Part model, mm, in its own coordinate system. A direction names the side the tool comes from. Coordinates: 2 decimals unless noted, no trailing zeros. Write each loop counter-clockwise with the first axis right and the second up, starting at its lowest first coordinate (ties: lowest second). Pieces come first, ordered by that corner, then holes. Notation, with made-up numbers: (56.5, -30.5) -> (104.5, -30.5) arc R28 cw to (104.5, -10.5) -> close; hole circle Ø10 at (51.25, 7.5). An arc over 180 degrees is marked (long way). Write item = value, one per line. Start each with the question number.
Q1. Band-saw the part on D-D, the plane x = 38.1. List the corners of the cut face in (y, z).
Q2. Tool access for faces 1 (the flat face through (25, 0, 17.462)), 2 (the flat face through (25, 0, 19.05)): list every direction of +Z, -Z, +X, -X, +Y, -Y with a clear straight run to the whole face (end or side of a thin tool).
Q3. Band-saw the part on B-B, the plane y = 3.25. List the corners of the cut face in (x, z), plus the area to 3 significant figures.
Q4. Band-saw the part on A-A, the plane z = 13. List the corners of the cut face in (x, y).
Q5. Probe line 1 (Y direction, x = 13.5, z = -15); line 2 (Z direction, x = 30.5, y = 0); line 3 (Z direction, x = 38.1, y = 12.05). List the from-to ranges inside material, lowest first.
Q6. Band-saw the part on C-C, the plane x = 18. List the corners of the cut face in (y, z), plus the area to 3 significant figures.
Q7. Pull direction Z, two halves, no side cores. Call faces 3 (the flat face through (25, -12.7, 0)), 4 (the flat face through (25, 0, -17.462)), 5 (the flat face through (25, 0, -19.05)): released by +Z, released by -Z, zero draft, split by the parting line, or undercut.
Autodesk Inventor part; units mm, degrees
ref_plane "Work Plane3" through (0, 12.7, 0) normal (0, 1, 0) x (-1, 0, 0)
ref_plane "Start Plane" through (0, 0, 0) normal (1, 0, 0) x (0, 1, 0)
ref_plane "End Plane" through (50.8, 0, 0) normal (1, 0, 0) x (0, 1, 0)
ref_plane "Work Plane3" through (0, 12.7, 0) normal (0, 1, 0) x (-1, 0, 0)
ref_plane "Start Plane" through (0, 0, 0) normal (1, 0, 0) x (0, 1, 0)
ref_plane "End Plane" through (50.8, 0, 0) normal (1, 0, 0) x (0, 1, 0)
sketch "Sketch" plane through (0, 0, 0) normal (1, 0, 0) x (0, 1, 0)
  line L0 (-12.7, 19.05) -> (12.7, 19.05)
  line L1 (12.7, 19.05) -> (12.7, -19.05)
  line L2 (12.7, -19.05) -> (-12.7, -19.05)
  line L3 (-12.7, -19.05) -> (-12.7, 19.05)
  line L4 (-12.7, 19.05) -> (12.7, -19.05) construction
  line L5 (12.7, 19.05) -> (-12.7, -19.05) construction
  line L6 (-11.1125, 17.4625) -> (11.1125, 17.4625)
  line L7 (11.1125, 17.4625) -> (11.1125, -17.4625)
  line L8 (11.1125, -17.4625) -> (-11.1125, -17.4625)
  line L9 (-11.1125, -17.4625) -> (-11.1125, 17.4625)
  line L10 (-11.1125, 17.4625) -> (11.1125, -17.4625) construction
  line L11 (11.1125, 17.4625) -> (-11.1125, -17.4625) construction
  point P0 (0, 0)
  dimension "d0" = 38.1
  dimension "d1" = 25.4
  dimension "d2" = 1.5875
  dimension "d3" = 1.5875
extrude "Body" add sketch "Sketch" along normal up to surface (50.8 mm away) from surface at 0
sketch "Sketch8" plane through (0, 0, 0) normal (1, 0, 0) x (0, 1, 0)
  line L0 (0, 0) -> (10, 0)
ref_plane "Work Plane6" through (0, 0, 0) normal (0, 0, -1) x (0, 1, 0)
sketch "Sketch9" plane through (0, 0, 0) normal (0, 0, -1) x (0, 1, 0)
  line L0 (-17.78, 0) -> (17.78, 0)
  line L1 (-17.78, 50.8) -> (17.78, 50.8)
  dimension "d21" = 50.8
sketch "Sketch5" plane through (0, 12.7, -19.05) normal (0, 1, 0) x (1, 0, 0)
  line L0 (0, -38.1) -> (0, 0)
  point P0 (0, -19.05)
  point P1 (38.1, -19.05)
  dimension "d22" = 38.1
hole "Hole2" at (38.1, 12.7, 0) direction (0, -1, 0) diameter 11.1125 end through all
equation "\"d3\" = d2"
equation "\"G_OFFSET_START\" = 0"
equation "\"G_OFFSET_END\" = 0"
equation "\"d17\" = d4 + G_OFFSET_END"
equation "\"G_L\" = d21"
properties part number "1606067191933"
Ans:
q1.outline = (-12.7, -19.05) -> (12.7, -19.05) -> (12.7, -5.56) -> (11.11, -5.56) -> (11.11, -17.46) -> (-11.11, -17.46) -> (-11.11, -5.56) -> (-12.7, -5.56) -> close; (-12.7, 5.56) -> (-11.11, 5.56) -> (-11.11, 17.46) -> (11.11, 17.46) -> (11.11, 5.56) -> (12.7, 5.56) -> (12.7, 19.05) -> (-12.7, 19.05) -> close
q2.face_1 = +X, -X
q2.face_2 = +Z, +X, -X, +Y, -Y
q3.outline = (0, -19.05) -> (50.8, -19.05) -> (50.8, -17.46) -> (0, -17.46) -> close; (0, 17.46) -> (50.8, 17.46) -> (50.8, 19.05) -> (0, 19.05) -> close
q3.area = 161 mm2
q4.outline = (0, -12.7) -> (50.8, -12.7) -> (50.8, -11.11) -> (0, -11.11) -> close; (0, 11.11) -> (50.8, 11.11) -> (50.8, 12.7) -> (0, 12.7) -> close
q5.line_1 = -12.7 to -11.11, 11.11 to 12.7
q5.line_2 = -19.05 to -17.46, 17.46 to 19.05
q5.line_3 = -19.05 to -5.56, 5.56 to 19.05
q6.outline = (-12.7, -19.05) -> (12.7, -19.05) -> (12.7, 19.05) -> (-12.7, 19.05) -> close; hole (-11.11, -17.46) -> (11.11, -17.46) -> (11.11, 17.46) -> (-11.11, 17.46) -> close
q6.area = 192 mm2
q7.face_3 = zero draft
q7.face_4 = undercut
q7.face_5 = released by -Z
